Design review of the part built by this model. Coordinates are the model's own, in mm. Coordinates: 2 decimals unless noted, no trailing zeros. Write each loop counter-clockwise with the first axis right and the second up, starting at its lowest first coordinate (ties: lowest second). Pieces come first, ordered by that corner, then holes. Notation, with made-up numbers: (-25.5, 27) - (4.5, 27) arc R32 ccw to (4.5, 64) - close; hole circle Ø7 at (59.25, 1.25). An arc over 180 degrees is marked (long way). Answer as a JSON object with one key per item and string values.
Autodesk Inventor part; units mm, degrees
ref_plane "YZ Plane" through (0, 0, 0) normal (1, 0, 0) x (0, 1, 0)
ref_plane "XY Plane" through (0, 0, 0) normal (0, 0, 1) x (1, 0, 0)
ref_plane "工作平面1" through (0, 0, 1.5) normal (0, 0, -1) x (-1, 0, 0)
sketch "草圖1" plane through (0, 0, 0) normal (0, 0, 1) x (1, 0, 0)
  line L0 (0, 6) -> (0, -6)
  line L1 (0, -6) -> (-139, -6)
  line L2 (-139, -6) -> (-139, 6)
  line L3 (-149, 2) -> (-139, 2)
  line L4 (-139, 2) -> (-139, -2)
  line L5 (-139, -2) -> (-149, -2)
  line L6 (-149, -2) -> (-149, 2)
  line L7 (0, -9.6) -> (0, 15.6)
  line L8 (-148, -2) -> (-139, -2)
  line L9 (-139, -2) -> (-139, -6)
  line L10 (-139, 6) -> (-139, -2)
  line L11 (-139, -2) -> (-148, -2)
  line L12 (-139, 6) -> (0, 6)
  line L13 (139, -6) -> (139, 6)
  line L14 (139, 6) -> (139, -2)
  line L15 (139, -2) -> (139, -6)
  line L16 (139, -2) -> (148, -2)
  line L17 (149, 2) -> (139, 2)
  line L18 (148, -2) -> (139, -2)
  line L19 (139, -2) -> (149, -2)
  line L20 (149, -2) -> (149, 2)
  line L21 (139, 2) -> (139, -2)
  line L22 (0, -6) -> (139, -6)
  line L23 (139, 6) -> (0, 6)
  point P0 (0, 0)
  point P1 (0, 0)
  point P2 (0, 0)
  point P3 (-139, 6)
  point P4 (-139, -2)
  point P5 (-148, 2)
  point P6 (139, -2)
  point P7 (139, 6)
  point P8 (139, 6)
  point P9 (139, -2)
  point P10 (139, -2)
  dimension "d0" = 10
  dimension "d1" = 139
  dimension "d2" = 4
  dimension "d6" = 6
  dimension "d7" = 6
  dimension "d8" = 8
  dimension "d9" = 4
  dimension "d14" = 12
extrude "擠出1" add sketch "草圖1" along normal blind 3
ref_plane "工作平面1" through (0, 0, 1.5) normal (0, 0, -1) x (-1, 0, 0)
sketch "草圖3" plane through (0, 0, 3) normal (0, 0, 1) x (1, 0, 0)
  line L0 (0, 1.45) -> (-139, 1.45)
  line L1 (-139, 1.45) -> (-139, -1.45)
  line L2 (-139, -1.45) -> (0, -1.45)
  line L3 (0, -1.45) -> (0, 1.45)
  line L4 (-139, -2) -> (-139, -6)
  line L5 (-139, 6) -> (-139, 2)
  line L6 (-149, -2) -> (-139, -2)
  line L7 (-139, 2) -> (-149, 2)
  line L8 (-149, 2) -> (-149, -2)
  line L9 (-149, -2) -> (-139, -2)
  line L10 (-139, -2) -> (-139, 2)
  point P0 (0, 0)
  point P1 (0, 0)
  dimension "d15" = 2.9
extrude "擠出3" cut sketch "草圖3" against normal blind 10
equation "\"d9\" = -0.5 * d2 + 0.5 * d14"
properties part number "rod_5"
(1) For pin 1 (0.9 mm diameter, centred on x = 145.5, z = 1.5, fed in from +Y); pin 2 (1.5 mm diameter, centred on x = 146.5, z = 1.5, fed in from -Y); pin 3 (1.4 mm diameter, centred on y = 0, z = 1.5, fed in from -X), all flat-tipped, find the tip position at first contact; note any pin that passes through.
Solved:
{"pin 1": "stops at y = 2", "pin 2": "stops at y = -2", "pin 3": "stops at x = 0"}
(2) Take a section at B-B, the plane z = 1.6. Write out the cut boundary in (x, y).
Solved:
{"outline": "(-139, -6) - (139, -6) - (139, -2) - (149, -2) - (149, 2) - (139, 2) - (139, 6) - (-139, 6) - (-139, 1.45) - (0, 1.45) - (0, -1.45) - (-139, -1.45) - close"}
(3) To check wall thickness, follow line 1 (Y direction, x = -49, z = 1.2); line 2 (X direction, y = 3, z = 1.55); line 3 (X direction, y = 0.5, z = 2.5). State the ranges of each line that lie inside material, in increasing order. Write a range as from..to.
Solved:
{"line 1": "y = -6..-1.45, 1.45..6", "line 2": "x = -139..139", "line 3": "x = 0..149"}
(4) Take a section at A-A, the plane x = -51.5. Write out the cut boundary in (y, z).
Solved:
{"outline": "(-6, 0) - (-1.45, 0) - (-1.45, 3) - (-6, 3) - close; (1.45, 0) - (6, 0) - (6, 3) - (1.45, 3) - close"}
